Design review of the part built by this model. Coordinates are the model's own, in mm. Face numbers are marked on the shaded views. Give positions to 0.01 mm unless a question says otherwise; leave off trailing zeros. Order: outer loops, then holes, each group sorted by start corner. A loop starts at its lowest first (then second) coordinate and runs counter-clockwise, first axis right, second up. Notation, with made-up numbers: M 63,-11.75 L 89,-11.75 A17 cw 89,11.25 Z; hole C 13,-8.75 d8. An arc over 180 degrees is marked long. Answer as a JSON object with one key per item and string values.
Autodesk Inventor part; units mm, degrees
ref_plane "YZ Plane" through (0, 0, 0) normal (1, 0, 0) x (0, 1, 0)
ref_plane "XZ Plane" through (0, 0, 0) normal (0, 1, 0) x (-1, 0, 0)
ref_plane "XY Plane" through (0, 0, 0) normal (0, 0, 1) x (1, 0, 0)
sketch "Sketch1" plane through (0, 0, 0) normal (0, 0, 1) x (1, 0, 0)
  line L0 (0, 0) -> (60, 0)
  line L1 (60, 0) -> (60, 60)
  line L2 (60, 60) -> (0, 60)
  line L3 (0, 60) -> (0, 0)
  line L4 (5, 55) -> (55, 55) construction
  line L5 (55, 55) -> (55, 5) construction
  line L6 (55, 5) -> (5, 5) construction
  line L7 (5, 5) -> (5, 55) construction
  circle A0 centre (5, 55) radius 2.2
  circle A1 centre (55, 55) radius 2.2
  circle A2 centre (55, 5) radius 2.2
  circle A3 centre (5, 5) radius 2.2
  line L8 (7.5, 42.5) -> (52.5, 42.5) construction
  line L9 (52.5, 42.5) -> (52.5, 17.5) construction
  line L10 (52.5, 17.5) -> (7.5, 17.5) construction
  line L11 (7.5, 17.5) -> (7.5, 42.5) construction
  circle A4 centre (7.5, 42.5) radius 5
  circle A5 centre (7.5, 42.5) radius 2.1
  dimension "d0" = 60
  dimension "d1" = 60
  dimension "d2" = 50
  dimension "d3" = 50
  dimension "d4" = 5
  dimension "d5" = 5
  dimension "d6" = 4.4
  dimension "d7" = 4.4
  dimension "d8" = 4.4
  dimension "d9" = 4.4
  dimension "d10" = 45
  dimension "d11" = 25
  dimension "d12" = 17.5
  dimension "d13" = 7.5
  dimension "d14" = 10
  dimension "d15" = 4.2
extrude "Extrusion1" add sketch "Sketch1" against normal blind 3 contours L3 L2 L1 L0 | A4 | A5
extrude "Extrusion2" add sketch "Sketch1" along normal blind 2 contours A4
fillet "Fillet1" radius 2 1 edges at (2.5, 42.5, 0)
extrude "Extrusion3" cut sketch "Sketch1" against normal through all contours A5
pattern_sketch "Sketch Driven Pattern1" of "Extrusion2", "Fillet1", "Extrusion3" from (7.5, 42.5, 0) copies at (52.5, 42.5, 0) at (52.5, 17.5, 0) at (7.5, 17.5, 0)
fillet "Fillet2" radius 5 4 edges at (0, 0, -1.5) (60, 0, -1.5) (60, 60, -1.5) (0, 60, -1.5)
equation "\"d4\" = -0.5 * d2 + 0.5 * d0"
equation "\"d5\" = -0.5 * d3 + 0.5 * d1"
equation "\"d12\" = -0.5 * d11 + 0.5 * d1"
equation "\"d13\" = -0.5 * d10 + 0.5 * d0"
properties part number "power_distribution_mount"
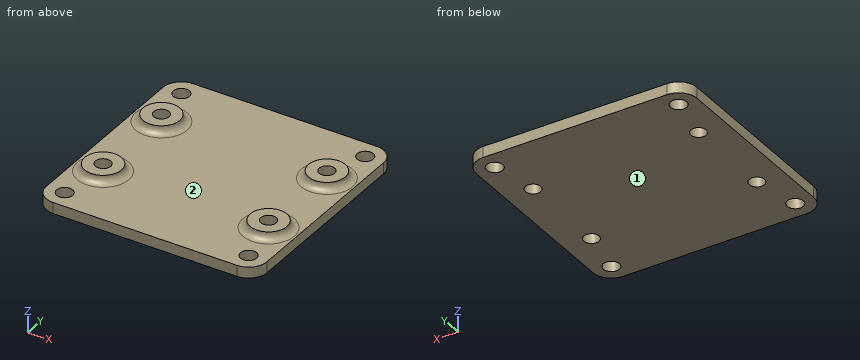
(1) We need section A-A (y = 17.5). Count the separate pieces of the cut face and the enclosed holes in it, plus the area to 3 significant figures.
Checked values:
{"separate pieces": "3", "enclosed holes": "0", "area": "181 mm^2"}
(2) To check wall thickness, follow L1, parallel to Y at x = 5, z = -1.35; L2, parallel to Y at x = 7.5, z = -0.4; L3, parallel to Y at x = 51, z = 0.35. State the ranges of each line that lie inside material, in increasing order. Write a range as from..to.
Checked values:
{"L1": "y = 0..2.8, 7.2..52.8, 57.2..60", "L2": "y = 0..15.4, 19.6..40.4, 44.6..60", "L3": "y = 11.83..16.03, 18.97..23.17, 36.83..41.03, 43.97..48.17"}
(3) We need section C-C (x = 27.5). Write out the cut boundary in (y, z).
Checked values:
{"outline": "M 0,-3 L 60,-3 L 60,0 L 0,0 Z"}
(4) We need section D-D (y = 4). Write out the cut boundary in (x, z).
Checked values:
{"outline": "M 0.1,-3 L 3.04,-3 L 3.04,0 L 0.1,0 Z; M 6.96,-3 L 53.04,-3 L 53.04,0 L 6.96,0 Z; M 56.96,-3 L 59.9,-3 L 59.9,0 L 56.96,0 Z"}
(5) Draft analysis for pull direction X (two halves, no side actions). For the marked faces 1 and 2, state which applies: +X half, -X half, draft (parallel to the pull), parting line (faces both ways), or undercut.
Checked values:
{"face 1": "draft", "face 2": "undercut"}
(6) We need section B-B (z = 0.9). Write out the cut boundary in (x, y).
Checked values:
{"outline": "C 7.5,17.5 d10.66; C 7.5,42.5 d10.66; C 52.5,17.5 d10.66; C 52.5,42.5 d10.66; hole C 7.5,17.5 d4.2; hole C 7.5,42.5 d4.2; hole C 52.5,17.5 d4.2; hole C 52.5,42.5 d4.2"}
(7) Insertion check: pin 1 (5.5 mm diameter, centred on x = 55, y = 55, fed in from -Z); pin 2 (7 mm diameter, centred on x = 55, y = 5, fed in from +Z). Each pin has a flat end and moves straight along its axis. Give the tip position at first contact, or say it passes through.
Checked values:
{"pin 1": "stops at z = -3", "pin 2": "stops at z = 0"}
